from build123d import *

# Parameters (mm, degrees)
ESQUISSE2_R             = 3
ENL_V_MAT_EXTRU_2_DEPTH = 9
CONG_1_R                = 1


with BuildPart() as part:
    # Esquisse1 → Révolution1 (revolve)
    with BuildSketch(Plane.XY):
        Polygon((-3, 31), (-5, 31), (-5, 36), (5, 36), (5, 31), (3, 31), (3, 0), (-3, 0), align=None)
    revolve(axis=Axis((-3, 0, 0), (1, 0, 0)))

    # Esquisse2 → Enlèv. mat.-Extru.2 (cut, through all)
    with BuildSketch(Plane(origin=(3, 0, 0), x_dir=(0, 0, -1), z_dir=(1, 0, 0))):
        Circle(ESQUISSE2_R)
    extrude(amount=-ENL_V_MAT_EXTRU_2_DEPTH, mode=Mode.SUBTRACT)

    # Congé1
    cong_1_edges = [part.edges().sort_by_distance(p)[0] for p in [
        (-3, -31, 0),
        (3, -31, 0),
    ]]
    fillet(cong_1_edges, radius=CONG_1_R)


solid = part.part
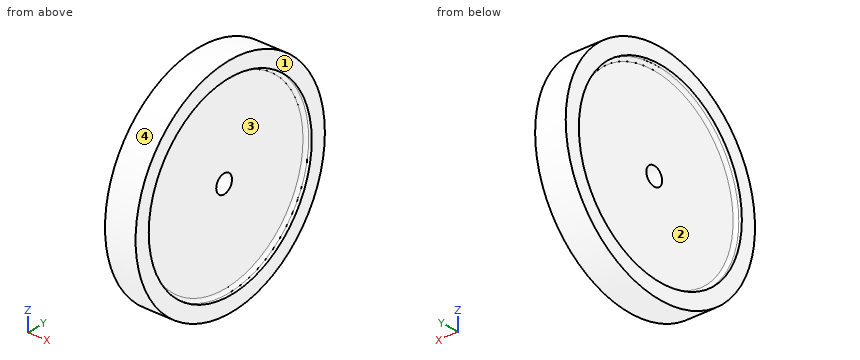
Could you check a few things on this model? Use its own coordinates, in mm. Face numbers are marked on the shaded views. Coordinates: 2 decimals unless noted, no trailing zeros. Loops run counter-clockwise (first coordinate to the right, second up) from the corner with the lowest first, then second, coordinate; pieces in that order, holes last. Notation, with made-up numbers: (-3, 53.5) -> (8, 53.5) arc R15 ccw to (8, 67.5) -> close; hole circle Ø5 at (-6, 18). An arc over 180 degrees is marked (long way). Answer in a Markdown table with one row per item.
(1) Imagine slicing it at A-A (y = 0). List the corners of the cut face in (x, z) for me.
Results found:
| item | result |
|---|---|
| outline | (-5, -36) -> (5, -36) -> (5, -31) -> (4, -31) arc R1 cw to (3, -30) -> (3, -3) -> (-3, -3) -> (-3, -30) arc R1 cw to (-4, -31) -> (-5, -31) -> close; (-5, 31) -> (-4, 31) arc R1 cw to (-3, 30) -> (-3, 3) -> (3, 3) -> (3, 30) arc R1 cw to (4, 31) -> (5, 31) -> (5, 36) -> (-5, 36) -> close |
(2) Imagine slicing it at C-C (x = 0.25). List the corners of the cut face in (y, z) for me.
Results found:
| item | result |
|---|---|
| outline | circle Ø72 at (0, 0); hole circle Ø6 at (0, 0) |
(3) If I drill on probe 1 along Z at (x, y) = (-4.6, 0); probe 2 along Z at (x, y) = (-3.5, 15); probe 3 along X at (y, z) = (-13.5, -1.5), over which ranges is the centre line in solid material (lowest first)?
Results found:
| item | result |
|---|---|
| probe 1 | z = -36 to -31, 31 to 36 |
| probe 2 | z = -32.73 to -26.98, 26.98 to 32.73 |
| probe 3 | x = -3 to 3 |
(4) Thinking about a two-plate mould opening in Z: for the marked faces 1, 2, 3 and 4, which applies, released by +Z, released by -Z, zero draft, split by the parting line, or undercut?
Results found:
| item | result |
|---|---|
| face 1 | zero draft |
| face 2 | undercut |
| face 3 | undercut |
| face 4 | split by the parting line |
(5) Will these pins go through, and if not, where does the flat tip stop? pin 1 Ø1 at (x, z) = (0.5, 8) entering from -Y; pin 2 Ø8 at (y, z) = (0, 0) entering from +X; pin 3 Ø4 at (y, z) = (23.5, -6) entering from -X.
Results found:
| item | result |
|---|---|
| pin 1 | stops at y = -35.21 |
| pin 2 | stops at x = 3 |
| pin 3 | stops at x = -3 |
